```python
from build123d import *

# Parameters (mm, degrees)
CROQUIS1_W              = 60.8
CROQUIS1_H              = 35.4
CROQUIS1_R              = 2.45
SALIENTE_EXTRUIR1_DEPTH = 2.5
REDONDEO1_R             = 2


with BuildPart() as part:
    # Croquis1 → Saliente-Extruir1 (new body)
    with BuildSketch(Plane(origin=(0, 0, 0), x_dir=(1, 0, 0), z_dir=(0, 1, 0))):
        Rectangle(CROQUIS1_W, CROQUIS1_H)
        with Locations(Location((-25.4, 12.7, 0), (0, 0, 270))):
            Circle(CROQUIS1_R, mode=Mode.SUBTRACT)
        with Locations(Location((-25.4, 0, 0), (0, 0, 270))):
            Circle(CROQUIS1_R, mode=Mode.SUBTRACT)
        with Locations(Location((-25.4, -12.7, 0), (0, 0, 270))):
            Circle(CROQUIS1_R, mode=Mode.SUBTRACT)
        with Locations(Location((25.4, -12.7, 0), (0, 0, 90))):
            Circle(CROQUIS1_R, mode=Mode.SUBTRACT)
        with Locations(Location((25.4, 0, 0), (0, 0, 90))):
            Circle(CROQUIS1_R, mode=Mode.SUBTRACT)
        with Locations(Location((25.4, 12.7, 0), (0, 0, 90))):
            Circle(CROQUIS1_R, mode=Mode.SUBTRACT)
    extrude(amount=SALIENTE_EXTRUIR1_DEPTH)

    # Redondeo1
    redondeo1_edges = [part.edges().sort_by_distance(p)[0] for p in [
        (30.4, 1.25, 17.7),
        (-30.4, 1.25, 17.7),
        (-30.4, 1.25, -17.7),
        (30.4, 1.25, -17.7),
    ]]
    fillet(redondeo1_edges, radius=REDONDEO1_R)


solid = part.part
```
Verification items for the finished model (mm, model axes). Coordinates: 2 decimals unless noted, no trailing zeros. Loops run counter-clockwise (first coordinate to the right, second up) from the corner with the lowest first, then second, coordinate; pieces in that order, holes last. Notation, with made-up numbers: (25.5, -12.75) - (41.5, -12.75) arc R12 cw to (41.5, -7.75) - close; hole circle Ø1 at (-18.75, 23.25). An arc over 180 degrees is marked (long way). Put each result on its own line as item: value.
Item 1: Section check C-C (x = 25.4). Enter the section's corners in (y, z).
Conclusion:
outline: (0, -17.7) - (2.5, -17.7) - (2.5, -15.15) - (0, -15.15) - close; (0, -10.25) - (2.5, -10.25) - (2.5, -2.45) - (0, -2.45) - close; (0, 2.45) - (2.5, 2.45) - (2.5, 10.25) - (0, 10.25) - close; (0, 15.15) - (2.5, 15.15) - (2.5, 17.7) - (0, 17.7) - close
Item 2: Section check A-A (y = 1.35). Enter the section's corners in (x, z), then the cut area to 3 significant figures.
Conclusion:
outline: (-30.4, -15.7) arc R2 ccw to (-28.4, -17.7) - (28.4, -17.7) arc R2 ccw to (30.4, -15.7) - (30.4, 15.7) arc R2 ccw to (28.4, 17.7) - (-28.4, 17.7) arc R2 ccw to (-30.4, 15.7) - close; hole circle Ø4.9 at (-25.4, -12.7); hole circle Ø4.9 at (-25.4, 0); hole circle Ø4.9 at (-25.4, 12.7); hole circle Ø4.9 at (25.4, -12.7); hole circle Ø4.9 at (25.4, 0); hole circle Ø4.9 at (25.4, 12.7)
area: 2,040 mm2
Item 3: Gauge pin test, flat ends, axial feed: pin 1 Ø3 at (x, z) = (-18.5, -4) entering from -Y; pin 2 Ø4 at (x, z) = (-25.4, 12.7) entering from +Y. Record the tip position at first contact, or that the pin passes through.
Conclusion:
pin 1: stops at y = 0
pin 2: passes through
Item 4: Draft check along X on faces 1 (the face through (-29.83, 1.27, 17.1)), 2 (the face through (22.97, 1.23, 0.32)), 3 (the face through (29.8, 1.27, 17.13)). Enter one of: pulls with the +X half, pulls with the -X half, needs draft (parallel to the pull), parting line crosses it, or undercut.
Conclusion:
face 1: pulls with the -X half
face 2: undercut
face 3: pulls with the +X half
Item 5: Section check B-B (z = -12.7). Enter the section's corners in (x, y), then the cut area to 4 significant figures.
Conclusion:
outline: (-30.4, 0) - (-27.85, 0) - (-27.85, 2.5) - (-30.4, 2.5) - close; (-22.95, 0) - (22.95, 0) - (22.95, 2.5) - (-22.95, 2.5) - close; (27.85, 0) - (30.4, 0) - (30.4, 2.5) - (27.85, 2.5) - close
area: 127.5 mm2
Item 6: Scan lines: line 1 along Z through (x, y) = (25.4, 1.25); line 2 along X through (y, z) = (1.3, 12.5); line 3 along Z through (x, y) = (-27, 0.85). Record each from-to range of solid material in increasing order.
Conclusion:
line 1: z = -17.7 to -15.15, -10.25 to -2.45, 2.45 to 10.25, 15.15 to 17.7
line 2: x = -30.4 to -27.84, -22.96 to 22.96, 27.84 to 30.4
line 3: z = -17.7 to -14.56, -10.84 to -1.86, 1.86 to 10.84, 14.56 to 17.7
Item 7: Section check D-D (z = 1). Enter the section's corners in (x, y), then the cut area to 3 significant figures.
Conclusion:
outline: (-30.4, 0) - (-27.64, 0) - (-27.64, 2.5) - (-30.4, 2.5) - close; (-23.16, 0) - (23.16, 0) - (23.16, 2.5) - (-23.16, 2.5) - close; (27.64, 0) - (30.4, 0) - (30.4, 2.5) - (27.64, 2.5) - close
area: 130 mm2
